Build history of the part. All positions in model axes, mm. A direction names the side the tool comes from. Round coordinates to 2 decimals unless told otherwise and drop trailing zeros. Order: outer loops, then holes, each group sorted by start corner. A loop starts at its lowest first (then second) coordinate and runs counter-clockwise, first axis right, second up. Notation, with made-up numbers: (-12, 81) -> (-6, 81) arc R18 ccw to (-6, 115) -> close; hole circle Ø8 at (31.5, 72.5). An arc over 180 degrees is marked (long way). Use a Markdown table: item, result. Add a question column.
Item 1: Slice it at B-B, the plane z = -35. Give the cut face in (x, y).
Item 2: Slice it at D-D, the plane z = 89. Give the cut face in (x, y).
Item 3: Pin check, flat tips, straight feed: pin 1 (4 mm diameter, centred on x = 61, z = 78, fed in from -Y); pin 2 (6 mm diameter, centred on y = 43, z = 101, fed in from -X); pin 3 (1.5 mm diameter, centred on x = 72.5, y = -6.5, fed in from +Z). Stop position of each tip, or through.
Item 4: 3-axis set-ups, long thin cutter, end or side, ignore diameter. For faces 1 (the face through (0, -1, 51)), 2 (the face through (197.5, -3, 75)), 3 (the face through (167, 90, -40)): which of +Z, -Z, +X, -X, +Y, -Y reach the whole face in a straight line?
Item 5: Slice it at A-A, the plane x = 100. Give the cut face in (y, z), plus the area to 3 significant figures.
Item 6: Two-plate mould, pull along Y, no slides. Class faces 4 (the face through (100, -100, -46)), 5 (the face through (149.184, -1.26, -31.925)), 6 (the face through (200, -1, 48)): released by +Y, released by -Y, zero draft, split by the parting line, or undercut.
Item 7: Probe L1, parallel to X at y = 55, z = 5; L2, parallel to Z at x = 100, y = 99.1; L3, parallel to X at y = -61, z = -29.5. List the from-to ranges inside material, lowest first.
Item 8: Slice it at C-C, the plane y = 45.5. Give the cut face in (x, z).
from build123d import *

# Parameters (mm, degrees)
F1_DEPTH     = 100
F2_T         = -2.5
F3_R         = 5
F4_DEPTH     = 200.001
F6_DEPTH     = 200
F7_T         = 10
F7_T3_DEPTH  = 168.4060893131
F7_T5_DEPTH  = 121.7259809119
F7_T7_DEPTH  = 121.7259809119
F7_T9_DEPTH  = 217.5
F7_T12_ANGLE = 49.9194838504


# Not quite as in the source:
# - a shell that OpenCascade refuses in one call is made with other operations: the cavity is built on its own and cut out


with BuildPart() as f1:
    # F0 (on Front) → F1 (new body, symmetric)
    with BuildSketch(Plane.XZ):
        with BuildLine():
            Line((200, 150), (0, 150))
            Line((0, 150), (0, 0))
            Line((0, 0), (93.6702797046, -43.5990676512))
            ThreePointArc((93.6702797046, -43.5990676512), (91.9360618935, -17.3519605387), (115, -30))
            ThreePointArc((115, -30), (112.6480394613, -38.0639381065), (106.3297202954, -43.5990676512))
            Line((106.3297202954, -43.5990676512), (200, 0))
            Line((200, 0), (200, 150))
        make_face()
        with BuildLine():
            ThreePointArc((115, -30), (91.9360618935, -17.3519605387), (93.6702797046, -43.5990676512))
            ThreePointArc((93.6702797046, -43.5990676512), (100, -45), (106.3297202954, -43.5990676512))
            ThreePointArc((106.3297202954, -43.5990676512), (112.6480394613, -38.0639381065), (115, -30))
        make_face()
    extrude(amount=F1_DEPTH, both=True)

    # F2
    f2_openings = [f1.faces().sort_by_distance(p)[0] for p in [
        (100, -100, 62.86367),
        (100, 0, 150),
    ]]
    offset(amount=F2_T, openings=f2_openings)

    # F3 (on face) → F4 (cut, through all)
    with BuildSketch(Plane(origin=(0, 100, 0), x_dir=(-1, 0, 0), z_dir=(0, 1, 0))):
        with Locations((-100, -35)):
            Circle(F3_R)
    extrude(amount=-F4_DEPTH, mode=Mode.SUBTRACT)

    # F5 (on face) → F6 (join)
    with BuildSketch(Plane.XZ.offset(100)):
        with BuildLine():
            Line((93.6702797046, -43.5990676512), (0, 0))
            Line((0, 0), (0, -50.5793318152))
            Line((0, -50.5793318152), (200, -50.5793318152))
            Line((200, -50.5793318152), (200, 0))
            Line((200, 0), (106.3297202954, -43.5990676512))
            ThreePointArc((106.3297202954, -43.5990676512), (103.2414491537, -44.64557979), (100, -45))
            ThreePointArc((100, -45), (96.7585508463, -44.64557979), (93.6702797046, -43.5990676512))
        make_face()
    extrude(amount=-F6_DEPTH)

    # F7: shell of thickness 10, made by hand


with BuildPart() as f7_core1:
    # F7_t2: copy of F1
    add(f1.part)

    # the walls: a layer under each face that stays
    f7_faces = [f7_core1.faces().sort_by_distance(p)[0] for p in [
        (200, 0, 49.7103340924),
        (100, 100, 49.7103340924),
        (105, 98.75, -35),
        (100, 97.5, 53.75),
        (100, -1.25, -42.5),
        (48.6126165436, -1.25, -19.8693228445),
        (151.3873834564, -1.25, -19.8693228445),
        (2.5, -1.25, 75.7969553435),
        (197.5, -1.25, 75.7969553435),
        (0, 0, 49.7103340924),
        (33.3333333333, -100, -17.1494431794),
        (31.25, 97.5308641975, 150),
    ]]
    thicken(f7_faces, amount=-F7_T, mode=Mode.SUBTRACT)

    # F7_s4 → F7_t3 (cut)
    with BuildSketch(Plane.XY.offset(-8.4060893131)):
        Polygon((197.4, 97.4), (197.5, 107.5), (207.5, 107.5), (207.5, 97.5), align=None)
        Polygon((2.6, 97.4), (2.5, 107.5), (-7.5, 107.5), (-7.5, 97.5), align=None)
    extrude(amount=F7_T3_DEPTH, mode=Mode.SUBTRACT)

    # F7_s6 → F7_t5 (cut)
    with BuildSketch(Plane(origin=(61.6500227345, 0, 28.695158383), x_dir=(0, 1, 0), z_dir=(0.9066045101, 0, 0.421981353))):
        Polygon((97.4, -81.7962706049), (107.5, -81.8962706049), (107.5, -91.8962706049), (97.5, -91.8962706049), align=None)
    extrude(amount=F7_T5_DEPTH, mode=Mode.SUBTRACT)

    # F7_s8 → F7_t7 (cut)
    with BuildSketch(Plane(origin=(-7.6209984834, 0, 3.547212942), x_dir=(0, 1, 0), z_dir=(0.9066045101, 0, -0.421981353))):
        Polygon((97.4, 2.6), (107.5, 2.5), (107.5, -7.5), (97.5, -7.5), align=None)
    extrude(amount=F7_T7_DEPTH, mode=Mode.SUBTRACT)

    # F7_s10 → F7_t9 (cut)
    with BuildSketch(Plane.XZ.offset(-107.5)):
        Polygon((2.6421981353, 1.6845711379), (-1.7198135302, -7.4721344139), (-7.5, -4.7817320608), (-7.5, 1.5939106869), align=None)
        Polygon((197.3578018647, 1.6845711379), (201.7198135302, -7.4721344139), (207.5, -4.7817320608), (207.5, 1.5939106869), align=None)
    extrude(amount=F7_T9_DEPTH, mode=Mode.SUBTRACT)

    # F7_s11 → F7_t12 (revolve, cut)
    with BuildSketch(Plane(origin=(93.6702797046, 0, -43.5990676512), x_dir=(0, 1, 0), z_dir=(-0.9066045101, 0, 0.421981353))):
        Polygon((97.4, -2.6), (107.5, -2.5), (107.5, 7.5), (97.5, 7.5), align=None)
    revolve(axis=Axis((100, 97.5, -30), (0, -1, 0)), revolution_arc=F7_T12_ANGLE, mode=Mode.SUBTRACT)


with BuildPart() as f1_1:
    add(f1.part)

    # what is left inside the walls is the cavity
    f7_cavity = [f7_core1.part.solids().sort_by_distance(p)[0] for p in [
        (149.789488, 30, -31.753537),
        (50.210512, 30, -31.753537),
    ]]
    add(f7_cavity, mode=Mode.SUBTRACT)


solid = f1_1.part
Check sheet entries:
| question | item | result |
|---|---|---|
| 1 | outline | (0, -100) -> (81.12, -100) -> (81.12, 97.5) -> (95, 97.5) -> (95, 100) -> (0, 100) -> close; (105, 97.5) -> (118.88, 97.5) -> (118.88, -100) -> (200, -100) -> (200, 100) -> (105, 100) -> close; hole (10, -90) -> (57.42, -90) -> (57.42, 90) -> (10, 90) -> close; hole (142.58, -90) -> (190, -90) -> (190, 90) -> (142.58, 90) -> close |
| 2 | outline | (0, -100) -> (2.5, -100) -> (2.5, 97.5) -> (197.5, 97.5) -> (197.5, -100) -> (200, -100) -> (200, 100) -> (0, 100) -> close |
| 3 | pin 1 | y = 97.5 |
| 3 | pin 2 | x = 0 |
| 3 | pin 3 | z = -30.64 |
| 4 | face 1 | +Z, -Z, -X, +Y, -Y |
| 4 | face 2 | +Z, -Y |
| 4 | face 3 | -Z |
| 5 | outline | (-100, -50.58) -> (100, -50.58) -> (100, -40) -> (97.5, -40) -> (97.5, -42.5) -> (-100, -42.5) -> close; (97.5, -30) -> (100, -30) -> (100, 150) -> (97.5, 150) -> close |
| 5 | area | 2,070 mm2 |
| 6 | face 4 | released by -Y |
| 6 | face 5 | undercut |
| 6 | face 6 | zero draft |
| 7 | L1 | 0 to 2.5, 197.5 to 200 |
| 7 | L2 | -50.58 to -40, -30 to 150 |
| 7 | L3 | 0 to 10, 45.61 to 69.3, 130.7 to 154.39, 190 to 200 |
| 8 | outline | (0, -50.58) -> (10, -50.58) -> (10, -12.93) -> (90.51, -50.4) arc R22.5 ccw to (90.9, -50.58) -> (109.1, -50.58) arc R22.5 ccw to (109.49, -50.4) -> (190, -12.93) -> (190, -50.58) -> (200, -50.58) -> (200, 150) -> (197.5, 150) -> (197.5, 1.59) -> (105.27, -41.33) arc R12.5 cw to (94.73, -41.33) -> (2.5, 1.59) -> (2.5, 150) -> (0, 150) -> close |
